Build history of the part. All positions in model axes, mm. Face numbers are marked on the shaded views. Round coordinates to 2 decimals unless told otherwise and drop trailing zeros. Write each loop counter-clockwise with the first axis right and the second up, starting at its lowest first coordinate (ties: lowest second). Pieces come first, ordered by that corner, then holes. Notation, with made-up numbers: (-1, 82) -> (28, 82) arc R9 ccw to (28, 90) -> close; hole circle Ø8 at (-34.5, -37.75). An arc over 180 degrees is marked (long way). Answer in a Markdown table with one row per item.
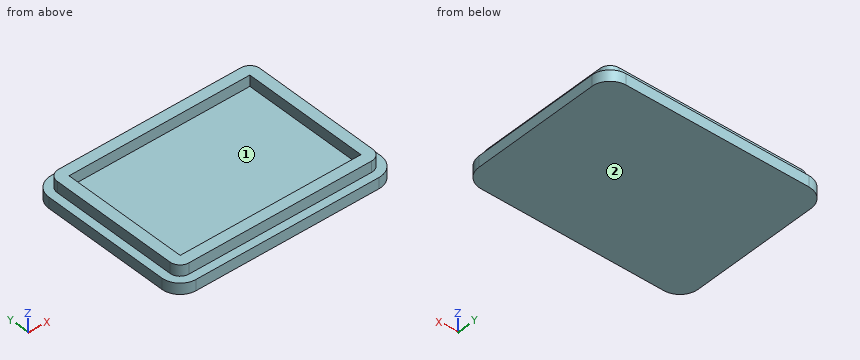
```python
from build123d import *

# Parameters (mm, degrees)
F1_DEPTH = 3
F3_DEPTH = 3
F4_T     = -3


with BuildPart() as f1:
    # F0 (on Top) → F1 (new body)
    with BuildSketch(Plane.XY):
        with BuildLine():
            Line((27.75, -17.5), (27.75, 17.5))
            ThreePointArc((27.75, 17.5), (26.9445436483, 19.4445436483), (25, 20.25))
            Line((25, 20.25), (-25, 20.25))
            ThreePointArc((-25, 20.25), (-26.9445436483, 19.4445436483), (-27.75, 17.5))
            Line((-27.75, 17.5), (-27.75, -17.5))
            ThreePointArc((-27.75, -17.5), (-26.9445436483, -19.4445436483), (-25, -20.25))
            Line((-25, -20.25), (25, -20.25))
            ThreePointArc((25, -20.25), (26.9445436483, -19.4445436483), (27.75, -17.5))
        make_face()
    extrude(amount=F1_DEPTH)

    # F2 (on Top) → F3 (join)
    with BuildSketch(Plane.XY):
        with BuildLine():
            Line((-25, -22.5), (10, -22.5))
            Line((10, -22.5), (25, -22.5))
            ThreePointArc((25, -22.5), (28.5355339059, -21.0355339059), (30, -17.5))
            Line((30, -17.5), (30, 17.5))
            ThreePointArc((30, 17.5), (28.5355339059, 21.0355339059), (25, 22.5))
            Line((25, 22.5), (-25, 22.5))
            ThreePointArc((-25, 22.5), (-28.5355339059, 21.0355339059), (-30, 17.5))
            Line((-30, 17.5), (-30, -17.5))
            ThreePointArc((-30, -17.5), (-28.5355339059, -21.0355339059), (-25, -22.5))
        make_face()
    extrude(amount=-F3_DEPTH)

    # F4
    f4_openings = [f1.faces().sort_by_distance(p)[0] for p in [
        (0, 0, 3),
    ]]
    offset(amount=F4_T, openings=f4_openings, kind=Kind.INTERSECTION)


solid = f1.part
```
Q1. Saw through at B-B on x = 16. Write the cut outline in (y, z).
A:
| item | result |
|---|---|
| outline | (-22.5, -3) -> (22.5, -3) -> (22.5, 0) -> (20.25, 0) -> (20.25, 3) -> (17.25, 3) -> (17.25, 0) -> (-17.25, 0) -> (-17.25, 3) -> (-20.25, 3) -> (-20.25, 0) -> (-22.5, 0) -> close |
Q2. Saw through at C-C on y = 5. Write the cut outline in (x, z).
A:
| item | result |
|---|---|
| outline | (-30, -3) -> (30, -3) -> (30, 0) -> (27.75, 0) -> (27.75, 3) -> (24.75, 3) -> (24.75, 0) -> (-24.75, 0) -> (-24.75, 3) -> (-27.75, 3) -> (-27.75, 0) -> (-30, 0) -> close |
Q3. Drop flat-ended pins along their axis: P1, Ø2.5, axis at y = 1.5, z = 1.5, coming from the +X side; P2, Ø1.5, axis at x = 0, y = 6.5, coming from the +Z side; P3, Ø1.5, axis at x = 3, z = 1.5, coming from the +Y side. Give the stop position or say it passes through.
A:
| item | result |
|---|---|
| P1 | x = 27.75 |
| P2 | z = 0 |
| P3 | y = 20.25 |
Q4. Two-plate mould, pull along X, no slides. Class the marked faces 1 and 2: released by +X, released by -X, zero draft, split by the parting line, or undercut.
A:
| item | result |
|---|---|
| face 1 | undercut |
| face 2 | zero draft |
Q5. Wall check: line 1 (Y direction, x = 22, z = 2.15); line 2 (X direction, y = -16, z = 0.55); line 3 (Z direction, x = 14, y = -6). Give the ranges that are in metal, low to high. Write a range as [from, to].
A:
| item | result |
|---|---|
| line 1 | [-20.25, -17.25], [17.25, 20.25] |
| line 2 | [-27.75, -24.75], [24.75, 27.75] |
| line 3 | [-3, 0] |
Q6. Saw through at D-D on x = 26. Write the cut outline in (y, z), plus the area to 3 significant figures.
A:
| item | result |
|---|---|
| outline | (-22.4, -3) -> (22.4, -3) -> (22.4, 0) -> (20.06, 0) -> (20.06, 3) -> (-20.06, 3) -> (-20.06, 0) -> (-22.4, 0) -> close |
| area | 255 mm² |
Q7. Saw through at A-A on z = 2.1. Write the cut outline in (x, y).
A:
| item | result |
|---|---|
| outline | (-27.75, -17.5) arc R2.75 ccw to (-25, -20.25) -> (25, -20.25) arc R2.75 ccw to (27.75, -17.5) -> (27.75, 17.5) arc R2.75 ccw to (25, 20.25) -> (-25, 20.25) arc R2.75 ccw to (-27.75, 17.5) -> close; hole (-24.75, -17.25) -> (24.75, -17.25) -> (24.75, 17.25) -> (-24.75, 17.25) -> close |
